Check sheet for the modelled part. Datum: model origin and axes. Units: mm. Coordinates: 2 decimals unless noted, no trailing zeros. Loops run counter-clockwise (first coordinate to the right, second up) from the corner with the lowest first, then second, coordinate; pieces in that order, holes last. Notation, with made-up numbers: M 70.25,46.25 L 97.25,46.25 A22 ccw 97.25,69.25 Z; hole C 57.5,10 d11. An arc over 180 degrees is marked long. Return JSON: item names as keys, results as strings.
from build123d import *

# Parameters (mm, degrees)
F0_W       = 115.6759760343
F0_H       = 74.756577611
F1_DEPTH   = 12.7
F2_R       = 9.4593135563
F3_DEPTH   = 25.4
F4_W       = 115.6759760343
F4_H       = 74.756577611
F4_R       = 8.4889409242
F5_DEPTH   = 25.4
F6_R       = 8.1100294651
F1_FACE1_W = 115.6759760343
F1_FACE1_H = 74.756577611
F7_DEPTH   = 25.4


with BuildPart() as f1:
    # F0 (on Front) → F1 (new body, symmetric)
    with BuildSketch(Plane.XZ):
        with Locations((2.7541879099, 0)):
            Rectangle(F0_W, F0_H)
    extrude(amount=F1_DEPTH, both=True)

    # F2 (on face) → F3 (join)
    with BuildSketch(Plane.XZ.offset(12.7)):
        with Locations((-30.2960947156, 18.0989615619)):
            Circle(F2_R)
    extrude(amount=-F3_DEPTH)

    # F4 (on face) → F5 (join)
    with BuildSketch(Plane(origin=(0, 12.7, 0), x_dir=(-1, 0, 0), z_dir=(0, 1, 0))):
        with Locations((-2.7541879099, 0)):
            Rectangle(F4_W, F4_H)
        with Locations((-43.9671128988, 24.5215520263)):
            Circle(F4_R, mode=Mode.SUBTRACT)
        with Locations((-43.9671128988, 24.5215520263)):
            Circle(F4_R)
    extrude(amount=-F5_DEPTH)

    # F6 (on Front) + F1_face1 (on face) → F7 (intersect)
    with BuildSketch(Plane.XZ):
        with Locations((37.1541380882, 23.0683349073)):
            Circle(F6_R)
    with BuildSketch(Plane(origin=(2.7541879099, 12.7, 0), x_dir=(1, 0, 0), z_dir=(0, 1, 0))):
        Rectangle(F1_FACE1_W, F1_FACE1_H)
    extrude(amount=-F7_DEPTH, dir=(0, -1, 0), mode=Mode.INTERSECT)


solid = f1.part
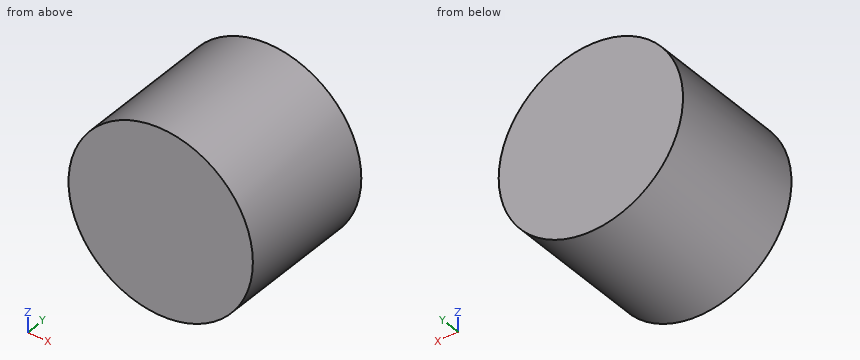
1) Section check A-A on x = 33.5. Record the cut outline in (y, z).
Answers:
{"outline": "M 0,15.83 L 12.7,15.83 L 12.7,30.31 L 0,30.31 Z"}
2) Scan lines: line 1 along Z through (x, y) = (39.75, 10.25); line 2 along Z through (x, y) = (30.25, 2.75); line 3 along X through (y, z) = (6.25, 29.5). Record each from-to range of solid material in increasing order. Write a range as [from, to].
Answers:
{"line 1": "[15.38, 30.75]", "line 2": "[18.81, 27.32]", "line 3": "[32.21, 42.09]"}
3) Section check B-B on y = 10.25. Record the cut outline in (x, z), then the cut area to 3 significant figures.
Answers:
{"outline": "C 37.15,23.07 d16.22", "area": "207 mm²"}
4) Go/stop test with flat-tipped pins: pin 1 Ø8 at (x, z) = (43.5, 22) entering from -Y; pin 2 Ø2 at (y, z) = (11, 17.5) entering from +X; pin 3 Ø4 at (x, y) = (34, 4) entering from -Z; pin 4 Ø1.5 at (x, y) = (36, 5.5) entering from +Z. Record where each tip stops, or that it passes through.
Answers:
{"pin 1": "y = 0", "pin 2": "x = 43.86", "pin 3": "z = 15.04", "pin 4": "z = 31.17"}
5) Section check C-C on z = 17.75. Record the cut outline in (x, y).
Answers:
{"outline": "M 31.03,0 L 43.28,0 L 43.28,12.7 L 31.03,12.7 Z"}
